Can you work these out from the model? Positions are in its coordinate system, mm. A direction names the side the tool comes from. Give positions to 0.01 mm unless a question says otherwise; leave off trailing zeros. Loops run counter-clockwise (first coordinate to the right, second up) from the corner with the lowest first, then second, coordinate; pieces in that order, holes last. Notation, with made-up numbers: (32, -10) - (65, -10) arc R22 cw to (65, 0) - close; hole circle Ø4 at (41.25, -15). An arc over 180 degrees is marked (long way). Answer as a JSON object with one key per item and string values.
Autodesk Inventor part; units mm, degrees
ref_plane "YZ Plane" through (0, 0, 0) normal (1, 0, 0) x (0, 1, 0)
ref_plane "XZ Plane" through (0, 0, 0) normal (0, 1, 0) x (-1, 0, 0)
ref_plane "XY Plane" through (0, 0, 0) normal (0, 0, 1) x (1, 0, 0)
sketch "Sketch1" plane through (0, 0, 0) normal (0, 1, 0) x (-1, 0, 0)
  line L0 (0, 0) -> (12.7, 0)
  line L1 (12.7, 0) -> (12.7, -47.625)
  line L2 (12.7, -47.625) -> (0, -47.625)
  line L3 (0, -47.625) -> (0, 0)
  line L4 (6.35, 0) -> (6.35, -6.35)
  circle A0 centre (6.35, -6.35) radius 2.1082
  line L5 (6.35, -6.35) -> (6.35, -19.05)
  circle A1 centre (6.35, -19.05) radius 2.1082
  line L6 (6.35, -19.05) -> (6.35, -53.975)
  line L7 (6.35, -53.975) -> (12.7, -53.975)
  circle A2 centre (12.7, -53.975) radius 2.1082
  line L8 (12.7, -53.975) -> (12.7, -60.325)
  arc A3 (12.7, -60.325) -> (12.7, -47.625) centre (12.7, -53.975) ccw
  line L9 (0, -47.625) -> (0, -53.975)
  line L10 (12.7, -60.325) -> (3.175, -60.325)
  line L11 (0, -57.15) -> (0, -53.975)
  arc A4 (0, -57.15) -> (3.175, -60.325) centre (3.175, -57.15) ccw
  dimension "d0" = 12.7
  dimension "d1" = 6.35
  dimension "d2" = 4.2164
  dimension "d3" = 47.625
  dimension "d4" = 12.7
  dimension "d5" = 34.925
  dimension "d6" = 6.35
  dimension "d7" = 4.2164
  dimension "d8" = 6.35
  dimension "d9" = 3.175
extrude "Extrusion1" add sketch "Sketch1" along normal blind 3.175 contours L0 L4 A0 L5 A1 L6 L2 L3 | L0 L1 L2 L6 A1 L5 A0 L4 | L2 L6 L7 A2 L8 L10 A4 L11 L9 | L2 A3 L8 A2 L7 L6
properties part number "wing mount no stopper" material "Aluminum 6061"
1) If we mould it in two halves opening along X, with no side actions, what happens to faces 1 (the flat face through (0, 2, -29)), 2 (the cylindrical face through (-6.08, 1.57, -8.44)), 3 (the flat face through (-8, 2, -60.325)), 4 (the cylindrical face through (-19.05, 1.57, -53.84))? For each: released by +X, released by -X, zero draft, split by the parting line, or undercut.
Check sheet entries:
{"face 1": "released by +X", "face 2": "undercut", "face 3": "zero draft", "face 4": "released by -X"}
2) Which directions (+Z, -Z, +X, -X, +Y, -Y) give clear straight access to the entire face, cutting with the end or side of a thin tool? Please do faces 5 (the flat face through (-12.7, 2, -23)), 6 (the cylindrical face through (-0.955, 1.565, -59.42)).
Check sheet entries:
{"face 5": "+Z, -X, +Y, -Y", "face 6": "-Z, +X, +Y, -Y"}
3) I need wall thicknesses on L1, parallel to Z at x = -6.35, y = 2.45 (3 decimals); L2, parallel to X at y = 2.3, z = -19.05; L3, parallel to Z at x = -5, y = 2.4 (3 decimals). Which ranges of each line are inside material? Lowest first, please.
Check sheet entries:
{"L1": "-60.325 to -21.158, -16.942 to -8.458, -4.242 to 0", "L2": "-12.7 to -8.46, -4.24 to 0", "L3": "-60.325 to -20.669, -17.431 to -7.969, -4.731 to 0"}
4) I'm going to push flat-ended pins straight in: P1, Ø5, axis at x = -6.35, z = -6.35, coming from the +Y side (3 decimals); P2, Ø1, axis at x = -16.5, y = 1.5, coming from the +Z side. Where does each tip first touch, or does it pass through?
Check sheet entries:
{"P1": "y = 3.175", "P2": "z = -48.55"}
5) Imagine slicing it at C-C on y = 1.3. Write out the boundary of the cut face in (x, z) (3 decimals).
Check sheet entries:
{"outline": "(-12.7, -60.325) - (-3.175, -60.325) arc R3.175 ccw to (0, -57.15) - (0, 0) - (-12.7, 0) - (-12.7, -47.625) arc R6.35 ccw to start; hole circle Ø4.216 at (-12.7, -53.975); hole circle Ø4.216 at (-6.35, -19.05); hole circle Ø4.216 at (-6.35, -6.35)"}
6) Imagine slicing it at B-B on x = -13.25. Write out the boundary of the cut face in (y, z) (3 decimals).
Check sheet entries:
{"outline": "(0, -60.301) - (3.175, -60.301) - (3.175, -56.01) - (0, -56.01) - close; (0, -51.94) - (3.175, -51.94) - (3.175, -47.649) - (0, -47.649) - close"}
7) Imagine slicing it at D-D on x = -7.25. Write out the boundary of the cut face in (y, z) (3 decimals).
Check sheet entries:
{"outline": "(0, -60.325) - (3.175, -60.325) - (3.175, -20.956) - (0, -20.956) - close; (0, -17.144) - (3.175, -17.144) - (3.175, -8.256) - (0, -8.256) - close; (0, -4.444) - (3.175, -4.444) - (3.175, 0) - (0, 0) - close"}
8) Imagine slicing it at A-A on z = -19.05. Write out the boundary of the cut face in (x, y) (3 decimals).
Check sheet entries:
{"outline": "(-12.7, 0) - (-8.458, 0) - (-8.458, 3.175) - (-12.7, 3.175) - close; (-4.242, 0) - (0, 0) - (0, 3.175) - (-4.242, 3.175) - close"}
